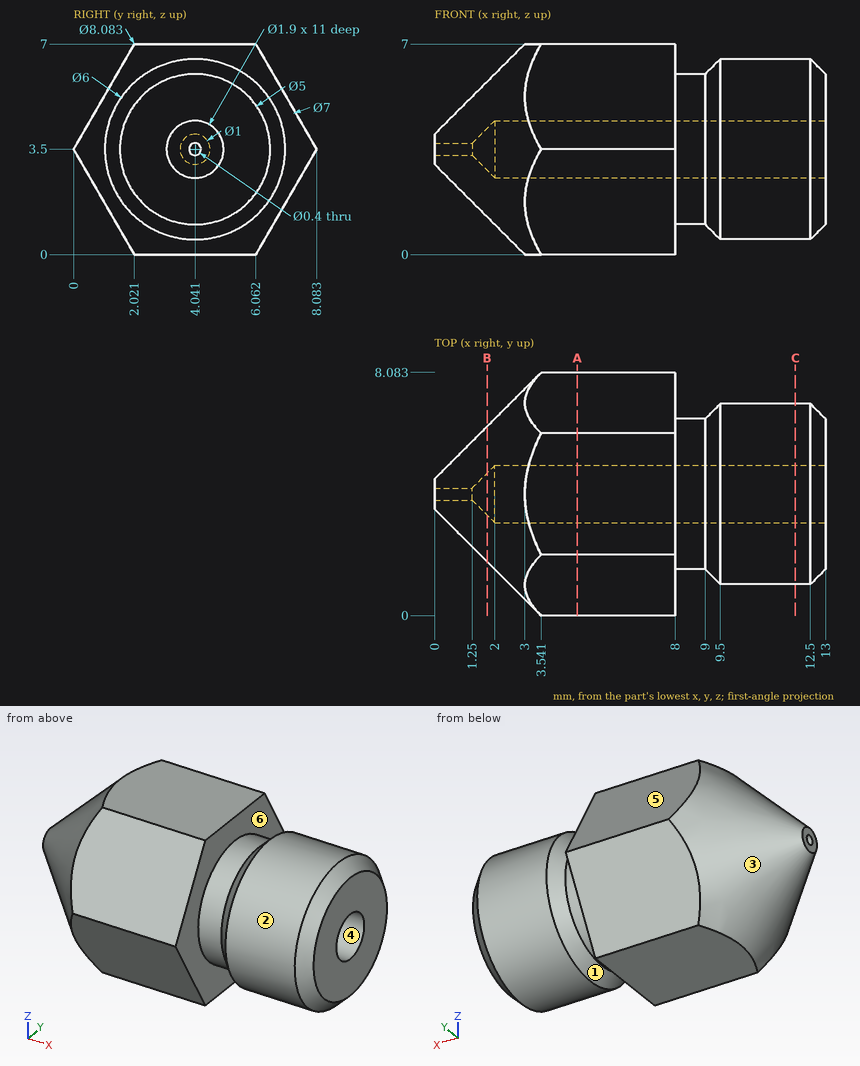
Geometry: see drawing. Coordinates: mm, zero at the bounding-box minimum. A direction names the side the tool comes from. Coordinates: 2 decimals unless noted, no trailing zeros. Order: outer loops, then holes, each group sorted by start corner. A loop starts at its lowest first (then second) coordinate and runs counter-clockwise, first axis right, second up. Notation, with made-up numbers: M 50,-30.5 L 85,-30.5 A9 cw 85,-20.5 Z; hole C 77.25,52 d7. An arc over 180 degrees is marked long. Write item = value, one per line. Start each with the question number.
(1) Section B-B on x = 1.75. Output: boundary loops of the cut face in (y, z).
(2) Section A-A on x = 4.75. Output: boundary loops of the cut face in (y, z), and give its area (3 significant figures).
(3) Pull-direction query (X, two-part tool) for the marked faces 1, 2 and 3; classes: released by +X, released by -X, zero draft, split by the parting line, or undercut.
(4) Section C-C on x = 12. Output: boundary loops of the cut face in (y, z).
(5) Line query: line 1 along Z through (x, y) = (3.5, 4.25); line 2 along X through (y, z) = (3.5, 0.5); line 3 along Y through (x, z) = (0.7, 3.5). Output: solid intervals per line, ascending. Write a range as [from, to].
(6) Reachability of the marked faces 4, 5 and 6 from +Z, -Z, +X, -X, +Y, -Y: full face, straight path, thin tool, end or side. Return the list, or none.
(7) First-contact query: P1, Ø2.5, axis at y = 3, z = 3, coming from the -X side; P2, Ø1.5, axis at y = 4.04, z = 3.5, coming from the +X side. Flat tips, straight axial feed; report the tip coordinate or a pass-through.
Result set:
q1.outline = C 4.04,3.5 d4.5; hole C 4.04,3.5 d1.4
q2.outline = M 0,3.5 L 2.02,0 L 6.06,0 L 8.08,3.5 L 6.06,7 L 2.02,7 Z; hole C 4.04,3.5 d1.9
q2.area = 39.6 mm²
q3.face_1 = undercut
q3.face_2 = zero draft
q3.face_3 = released by -X
q4.outline = C 4.04,3.5 d6; hole C 4.04,3.5 d1.9
q5.line_1 = [0, 2.57], [4.43, 7]
q5.line_2 = [2.55, 8]
q5.line_3 = [2.84, 3.84], [4.24, 5.24]
q6.face_4 = +X
q6.face_5 = +Z, +X, -X, +Y
q6.face_6 = none
q7.P1 = 0
q7.P2 = 1.8
